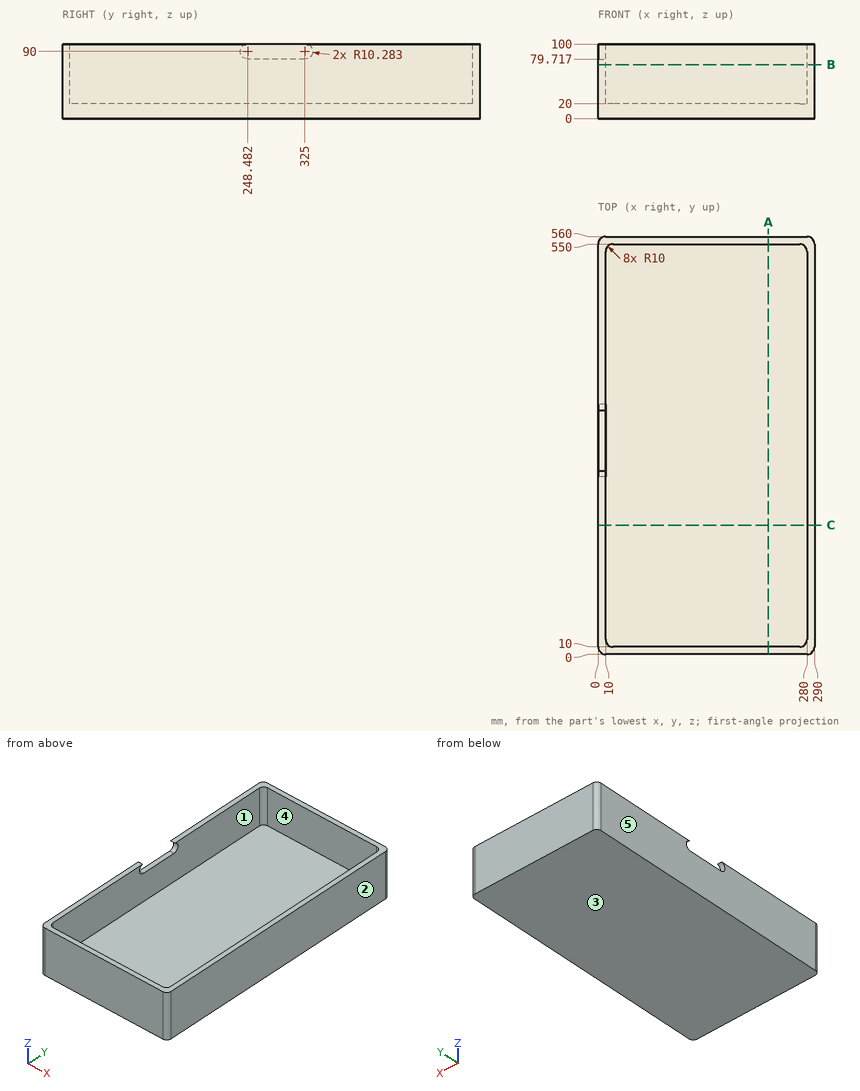
Study the drawing (mm; zero at the part's minimum x, y, z) and answer. A direction names the side the tool comes from. Round coordinates to 2 decimals unless told otherwise and drop trailing zeros. Write each loop counter-clockwise with the first axis right and the second up, starting at its lowest first coordinate (ties: lowest second). Pieces come first, ordered by that corner, then holes.
1) A cutting plane is placed at B-B on z = 72.5. Determine the outline of the cut face in (x, y), and give its area (3 significant figures).
2) Flat-ended cylindrical pins translate along their axes: P1, Ø4, axis at x = 195.5, y = 433.5, coming from the +Z side; P2, Ø3, axis at x = 7, y = 280, coming from the +Z side. Find the tip coordinate at first contact, or state that the pin passes through.
3) Determine the mould class of the marked faces 3, 4 and 5 for opening direction X: pulls with the +X half, pulls with the -X half, needs draft (parallel to the pull), parting line crosses it, or undercut.
4) A cutting plane is placed at A-A on x = 228. Determine the outline of the cut face in (y, z), and give its area (3 significant figures).
5) A cutting plane is placed at C-C on y = 173. Determine the outline of the cut face in (x, z), and give its area (3 significant figures).
6) Consider probe 1 along Y at (x, z) = (209, 33.5); probe 2 along X at (y, z) = (201.5, 20.5); probe 3 along Z at (x, y) = (168, 59.5). Determine where each line is inside the solid, lowest interval first.
7) Which of the six approach directions +Z, -Z, +X, -X, +Y, -Y give full straight-line access (tool end or side, diameter ignored) to the marked faces 1 and 2?
Entries:
1. outline: (0, 10) arc R10 ccw to (10, 0) - (280, 0) arc R10 ccw to (290, 10) - (290, 550) arc R10 ccw to (280, 560) - (10, 560) arc R10 ccw to (0, 550) - close; hole (10, 20) arc R10 ccw to (20, 10) - (270, 10) arc R10 ccw to (280, 20) - (280, 540) arc R10 ccw to (270, 550) - (20, 550) arc R10 ccw to (10, 540) - close
1. area: 16,600 mm2
2. P1: stops at z = 20
2. P2: stops at z = 79.72
3. face 3: needs draft
3. face 4: undercut
3. face 5: pulls with the -X half
4. outline: (0, 0) - (560, 0) - (560, 100) - (550, 100) - (550, 20) - (10, 20) - (10, 100) - (0, 100) - close
4. area: 12,800 mm2
5. outline: (0, 0) - (290, 0) - (290, 100) - (280, 100) - (280, 20) - (10, 20) - (10, 100) - (0, 100) - close
5. area: 7,400 mm2
6. probe 1: y = 0 to 10, 550 to 560
6. probe 2: x = 0 to 10, 280 to 290
6. probe 3: z = 0 to 20
7. face 1: +Z
7. face 2: +Z, -Z, +X, +Y, -Y
